Geometry check sheet. Reference: the model listing, model coordinates, mm. Coordinates: 2 decimals unless noted, no trailing zeros. Loops run counter-clockwise (first coordinate to the right, second up) from the corner with the lowest first, then second, coordinate; pieces in that order, holes last. Notation, with made-up numbers: M 40,24 L 50,24 A24 ccw 50,45 Z; hole C 86.25,7.5 d5. An arc over 180 degrees is marked long. One line per question, with ' | ' between items. Start each with the question number.
from build123d import *

# Parameters (mm, degrees)
SKETCH1_W         = 210
SKETCH1_H         = 210
SKETCH1_R         = 1.5
SKETCH1_R_2       = 6.1
SKETCH1_R_3       = 1.765
SKETCH1_W_2       = 2.2
SKETCH1_H_2       = 20.2
MAINEXTRUDE_DEPTH = 4
ROUNDEDCORNERS_R  = 10


with BuildPart() as part:
    # Sketch1 → MainExtrude (new body)
    with BuildSketch(Plane(origin=(0, 0, 0), x_dir=(1, 0, 0), z_dir=(0, 1, 0))):
        Rectangle(SKETCH1_W, SKETCH1_H)
        with Locations((-99.833273811, 99.833273811)):
            Circle(SKETCH1_R, mode=Mode.SUBTRACT)
        with Locations((-99.833273811, -99.833273811)):
            Circle(SKETCH1_R, mode=Mode.SUBTRACT)
        with Locations((99.833273811, -99.833273811)):
            Circle(SKETCH1_R, mode=Mode.SUBTRACT)
        with Locations((99.833273811, 99.833273811)):
            Circle(SKETCH1_R, mode=Mode.SUBTRACT)
        with Locations((67.333333333, -65.25)):
            Circle(SKETCH1_R_2, mode=Mode.SUBTRACT)
        with Locations((0, -65.25)):
            Circle(SKETCH1_R_2, mode=Mode.SUBTRACT)
        with Locations((-67.333333333, -65.25)):
            Circle(SKETCH1_R_2, mode=Mode.SUBTRACT)
        with Locations((-67.333333333, 22.25)):
            Circle(SKETCH1_R_2, mode=Mode.SUBTRACT)
        with Locations((0, 22.25)):
            Circle(SKETCH1_R_2, mode=Mode.SUBTRACT)
        with Locations((67.333333333, 22.25)):
            Circle(SKETCH1_R_2, mode=Mode.SUBTRACT)
        with Locations((-50.666666667, -71.5)):
            Circle(SKETCH1_R_3, mode=Mode.SUBTRACT)
        with Locations((-50.666666667, -94.5)):
            Circle(SKETCH1_R_3, mode=Mode.SUBTRACT)
        with Locations((-16.666666667, -94.5)):
            Circle(SKETCH1_R_3, mode=Mode.SUBTRACT)
        with Locations((-16.666666667, -71.5)):
            Circle(SKETCH1_R_3, mode=Mode.SUBTRACT)
        with Locations((16.666666667, -71.5)):
            Circle(SKETCH1_R_3, mode=Mode.SUBTRACT)
        with Locations((16.666666667, -94.5)):
            Circle(SKETCH1_R_3, mode=Mode.SUBTRACT)
        with Locations((50.666666667, -94.5)):
            Circle(SKETCH1_R_3, mode=Mode.SUBTRACT)
        with Locations((50.666666667, -71.5)):
            Circle(SKETCH1_R_3, mode=Mode.SUBTRACT)
        with Locations((-46.066666667, -83)):
            Rectangle(SKETCH1_W_2, SKETCH1_H_2, mode=Mode.SUBTRACT)
        with Locations((-39.866666667, -83)):
            Rectangle(SKETCH1_W_2, SKETCH1_H_2, mode=Mode.SUBTRACT)
        with Locations((-33.666666667, -83)):
            Rectangle(SKETCH1_W_2, SKETCH1_H_2, mode=Mode.SUBTRACT)
        with Locations((-27.466666667, -83)):
            Rectangle(SKETCH1_W_2, SKETCH1_H_2, mode=Mode.SUBTRACT)
        with Locations((-21.266666667, -83)):
            Rectangle(SKETCH1_W_2, SKETCH1_H_2, mode=Mode.SUBTRACT)
        with Locations((21.266666667, -83)):
            Rectangle(SKETCH1_W_2, SKETCH1_H_2, mode=Mode.SUBTRACT)
        with Locations((27.466666667, -83)):
            Rectangle(SKETCH1_W_2, SKETCH1_H_2, mode=Mode.SUBTRACT)
        with Locations((33.666666667, -83)):
            Rectangle(SKETCH1_W_2, SKETCH1_H_2, mode=Mode.SUBTRACT)
        with Locations((39.866666667, -83)):
            Rectangle(SKETCH1_W_2, SKETCH1_H_2, mode=Mode.SUBTRACT)
        with Locations((46.066666667, -83)):
            Rectangle(SKETCH1_W_2, SKETCH1_H_2, mode=Mode.SUBTRACT)
    extrude(amount=MAINEXTRUDE_DEPTH)

    # RoundedCorners
    roundedcorners_edges = [part.edges().sort_by_distance(p)[0] for p in [
        (-105, 2, 105),
        (-105, 2, -105),
        (105, 2, -105),
        (105, 2, 105),
    ]]
    fillet(roundedcorners_edges, radius=ROUNDEDCORNERS_R)


solid = part.part
1. Draft check along Z on faces 1 (the cylindrical face through (-71.83, 1.97, -26.37)), 2 (the cylindrical face through (101.99, 2.03, -102.15)), 3 (the cylindrical face through (101.99, 2.03, 102.15)), 4 (the cylindrical face through (3.279, 1.972, -27.394)). Enter one of: +Z half, -Z half, draft (parallel to the pull), parting line (faces both ways), or undercut.
2. Thickness scan on line 1 (X direction, y = 3.05, z = -22.25); line 2 (X direction, y = 0.8, z = 94.5); line 3 (Z direction, x = 28.5, y = 3.1). Record the ranges inside material, lowest first.
3. Sectioned sample at B-B (z = 88.5). State how many separate pieces and enclosed holes the cut face has, and give its area (3 significant figures).
4. Sectioned sample at A-A (z = -22.25). Record the cut outline in (x, y).
Result:
1) face 1: undercut | face 2: -Z half | face 3: +Z half | face 4: undercut
2) line 1: x = -105 to -73.43, -61.23 to -6.1, 6.1 to 61.23, 73.43 to 105 | line 2: x = -105 to -52.43, -48.9 to -18.43, -14.9 to 14.9, 18.43 to 48.9, 52.43 to 105 | line 3: z = -105 to 72.9, 93.1 to 105
3) separate pieces: 11 | enclosed holes: 0 | area: 752 mm2
4) outline: M -105,0 L -73.43,0 L -73.43,4 L -105,4 Z; M -61.23,0 L -6.1,0 L -6.1,4 L -61.23,4 Z; M 6.1,0 L 61.23,0 L 61.23,4 L 6.1,4 Z; M 73.43,0 L 105,0 L 105,4 L 73.43,4 Z
